```python
from build123d import *

# Parameters (mm, degrees)
F1_DEPTH = 57.15
F2_DEPTH = 3.175


# Not quite as in the source:
# - a feature names something its author has since deleted; it is built from what else it names


with BuildPart() as f1:
    # F0 (on Top) → F1 (new body)
    with BuildSketch(Plane.XY):
        with BuildLine():
            ThreePointArc((0, -73.025), (51.6364726961, -51.6364726961), (73.025, 0))
            ThreePointArc((73.025, 0), (51.6364726961, 51.6364726961), (0, 73.025))
            Line((0, 73.025), (0, 66.675))
            ThreePointArc((0, 66.675), (1.5879504187, 66.6560877825), (3.175, 66.5993618588))
            ThreePointArc((3.175, 66.5993618588), (6.220920948, 66.3841529852), (9.2537943589, 66.0297123647))
            ThreePointArc((9.2537943589, 66.0297123647), (50.3117896913, 43.752479279), (66.675, 0))
            ThreePointArc((66.675, 0), (50.3117896913, -43.752479279), (9.2537943589, -66.0297123647))
            ThreePointArc((9.2537943589, -66.0297123647), (6.220920948, -66.3841529852), (3.175, -66.5993618588))
            ThreePointArc((3.175, -66.5993618588), (1.5879504187, -66.6560877825), (0, -66.675))
            Line((0, -66.675), (0, -73.025))
        make_face()
        with BuildLine():
            Line((0, 66.675), (0, 73.025))
            ThreePointArc((0, 73.025), (-73.025, 0), (0, -73.025))
            Line((0, -73.025), (0, -66.675))
            ThreePointArc((0, -66.675), (-1.5879504187, -66.6560877825), (-3.175, -66.5993618588))
            ThreePointArc((-3.175, -66.5993618588), (-6.220920948, -66.3841529852), (-9.2537943589, -66.0297123647))
            ThreePointArc((-9.2537943589, -66.0297123647), (-66.675, 0), (-9.2537943589, 66.0297123647))
            ThreePointArc((-9.2537943589, 66.0297123647), (-6.220920948, 66.3841529852), (-3.175, 66.5993618588))
            ThreePointArc((-3.175, 66.5993618588), (-1.5879504187, 66.6560877825), (0, 66.675))
        make_face()
        with BuildLine():
            Line((-3.175, 57.15), (-3.175, 66.5993618588))
            ThreePointArc((-3.175, 66.5993618588), (-6.220920948, 66.3841529852), (-9.2537943589, 66.0297123647))
            ThreePointArc((-9.2537943589, 66.0297123647), (-4.840269288, 62.5305444087), (-3.175, 57.15))
        make_face()
        with BuildLine():
            ThreePointArc((9.2537943589, 66.0297123647), (6.220920948, 66.3841529852), (3.175, 66.5993618588))
            Line((3.175, 66.5993618588), (3.175, 57.15))
            ThreePointArc((3.175, 57.15), (4.840269288, 62.5305444087), (9.2537943589, 66.0297123647))
        make_face()
        with BuildLine():
            Line((3.175, -57.15), (3.175, -66.5993618588))
            ThreePointArc((3.175, -66.5993618588), (6.220920948, -66.3841529852), (9.2537943589, -66.0297123647))
            ThreePointArc((9.2537943589, -66.0297123647), (4.840269288, -62.5305444087), (3.175, -57.15))
        make_face()
        with BuildLine():
            ThreePointArc((-9.2537943589, -66.0297123647), (-6.220920948, -66.3841529852), (-3.175, -66.5993618588))
            Line((-3.175, -66.5993618588), (-3.175, -57.15))
            ThreePointArc((-3.175, -57.15), (-4.840269288, -62.5305444087), (-9.2537943589, -66.0297123647))
        make_face()
        with BuildLine():
            Line((0, -66.675), (0, 66.675))
            ThreePointArc((0, 66.675), (-1.5879504187, 66.6560877825), (-3.175, 66.5993618588))
            Line((-3.175, 66.5993618588), (-3.175, 57.15))
            Line((-3.175, 57.15), (-3.175, -57.15))
            Line((-3.175, -57.15), (-3.175, -66.5993618588))
            ThreePointArc((-3.175, -66.5993618588), (-1.5879504187, -66.6560877825), (0, -66.675))
        make_face()
        with BuildLine():
            ThreePointArc((3.175, 66.5993618588), (1.5879504187, 66.6560877825), (0, 66.675))
            Line((0, 66.675), (0, -66.675))
            ThreePointArc((0, -66.675), (1.5879504187, -66.6560877825), (3.175, -66.5993618588))
            Line((3.175, -66.5993618588), (3.175, -57.15))
            Line((3.175, -57.15), (3.175, 57.15))
            Line((3.175, 57.15), (3.175, 66.5993618588))
        make_face()
    extrude(amount=F1_DEPTH)

    # F0 (on Top) → F2 (join)
    with BuildSketch(Plane.XY):
        with BuildLine():
            ThreePointArc((-3.175, 57.15), (-4.840269288, 62.5305444087), (-9.2537943589, 66.0297123647))
            ThreePointArc((-9.2537943589, 66.0297123647), (-66.675, 0), (-9.2537943589, -66.0297123647))
            ThreePointArc((-9.2537943589, -66.0297123647), (-4.840269288, -62.5305444087), (-3.175, -57.15))
            Line((-3.175, -57.15), (-3.175, 57.15))
        make_face()
        with BuildLine():
            ThreePointArc((66.675, 0), (50.3117896913, 43.752479279), (9.2537943589, 66.0297123647))
            ThreePointArc((9.2537943589, 66.0297123647), (4.840269288, 62.5305444087), (3.175, 57.15))
            Line((3.175, 57.15), (3.175, -57.15))
            ThreePointArc((3.175, -57.15), (4.840269288, -62.5305444087), (9.2537943589, -66.0297123647))
            ThreePointArc((9.2537943589, -66.0297123647), (50.3117896913, -43.752479279), (66.675, 0))
        make_face()
    extrude(amount=F2_DEPTH)


solid = f1.part
```
Input: part model. Units: mm. Frame: model coordinates. A direction names the side the tool comes from. Give positions to 0.01 mm unless a question says otherwise; leave off trailing zeros. Order: outer loops, then holes, each group sorted by start corner. A loop starts at its lowest first (then second) coordinate and runs counter-clockwise, first axis right, second up. Notation, with made-up numbers: M -8.75,-25.5 L 25.25,-25.5 A23 cw 25.25,13.5 Z; hole C 85,32 d8. An arc over 180 degrees is marked long. Return JSON: item names as keys, results as strings.
Item 1: Access query for faces 1 (the cylindrical face through (-4.795, -62.464, 29.785)), 2 (the flat face through (-1, 1, 0)). Directions: +Z, -Z, +X, -X, +Y, -Y. A direction counts if a zero-diameter tool reaches every point of the face in a straight line with its end or side. Return the directions, or none.
Solutions:
{"face 1": "+Z", "face 2": "-Z, +X, -X, +Y, -Y"}
Item 2: Pull-direction query (X, two-part tool) for faces 3 (the flat face through (0, -5, 57.15)), 4 (the flat face through (-28, 1, 3.175)); classes: +X half, -X half, draft (parallel to the pull), parting line (faces both ways), or undercut.
Solutions:
{"face 3": "draft", "face 4": "undercut"}
Item 3: Cut plane C-C (x = -53). Return loops of the section in (y, z) (3 decimals).
Solutions:
{"outline": "M -50.236,0 L 50.236,0 L 50.236,57.15 L 40.454,57.15 L 40.454,3.175 L -40.454,3.175 L -40.454,57.15 L -50.236,57.15 Z"}
Item 4: Cut plane B-B (y = 22.5). Return loops of the section in (x, z) (3 decimals).
Solutions:
{"outline": "M -69.472,0 L 69.472,0 L 69.472,57.15 L 62.764,57.15 L 62.764,3.175 L 3.175,3.175 L 3.175,57.15 L -3.175,57.15 L -3.175,3.175 L -62.764,3.175 L -62.764,57.15 L -69.472,57.15 Z"}
Item 5: First-contact query: P1, Ø12, axis at y = -26.5, z = 17, coming from the -X side; P2, Ø4, axis at x = 12.5, z = 10.5, coming from the +Y side; P3, Ø2, axis at y = 54.5, z = 31, coming from the -X side. Flat tips, straight axial feed; report the tip coordinate or a pass-through.
Solutions:
{"P1": "x = -70.09", "P2": "y = 72.27", "P3": "x = -49.7"}
Item 6: Cut plane D-D (y = -20). Return loops of the section in (x, z) (3 decimals), then the cut area to 3 significant figures.
Solutions:
{"outline": "M -70.233,0 L 70.233,0 L 70.233,57.15 L 63.605,57.15 L 63.605,3.175 L 3.175,3.175 L 3.175,57.15 L -3.175,57.15 L -3.175,3.175 L -63.605,3.175 L -63.605,57.15 L -70.233,57.15 Z", "area": "1,500 mm^2"}
Item 7: Ray query, probe 1 along X at (y, z) = (26.5, 23) (3 decimals); probe 2 along X at (y, z) = (51.5, 21) (3 decimals); probe 3 along Z at (x, y) = (19.5, -13.5) (3 decimals). Return the intervals inside material, ascending.
Solutions:
{"probe 1": "-68.047 to -61.183, -3.175 to 3.175, 61.183 to 68.047", "probe 2": "-51.773 to -42.347, -3.175 to 3.175, 42.347 to 51.773", "probe 3": "0 to 3.175"}
Item 8: Cut plane A-A (z = 6.5). Return loops of the section in (x, y) (3 decimals).
Solutions:
{"outline": "C 0,0 d146.05; hole M -9.254,-66.03 A9.525 ccw -3.175,-57.15 L -3.175,57.15 A9.525 ccw -9.254,66.03 A66.675 ccw Z; hole M 3.175,-57.15 A9.525 ccw 9.254,-66.03 A66.675 ccw 9.254,66.03 A9.525 ccw 3.175,57.15 Z"}
